```python
from build123d import *

# Parameters (mm, degrees)
SKETCH1_R           = 4.1
BOSS_EXTRUDE1_DEPTH = 10
SKETCH2_W           = 28.190778624
SKETCH2_H           = 5
BOSS_EXTRUDE2_DEPTH = 15
SKETCH4_R           = 2.6
CUT_EXTRUDE1_DEPTH  = 20
CHAMFER1_SIZE       = 15
SKETCH5_R           = 5.5
CUT_EXTRUDE2_DEPTH  = 20


with BuildPart() as part:
    # Sketch1 → Boss-Extrude1 (new body)
    with BuildSketch(Plane.XY):
        Polygon((535.624793848, 194.951481696), (535.624793848, 0), (507.434015224, 0), (507.434015224, 184.690877396), (497.173410925, 212.881656019), (525.364189548, 223.142260319), align=None)
        with Locations((516.399102386, 203.916568858)):
            Circle(SKETCH1_R, mode=Mode.SUBTRACT)
    extrude(amount=BOSS_EXTRUDE1_DEPTH)

    # Sketch2 → Boss-Extrude2 (add)
    with BuildSketch(Plane.XY.offset(10)):
        with Locations((521.529404536, 2.5)):
            Rectangle(SKETCH2_W, SKETCH2_H)
    extrude(amount=BOSS_EXTRUDE2_DEPTH)

    # Sketch4 → Cut-Extrude1 (cut)
    with BuildSketch(Plane(origin=(0, 5, 0), x_dir=(1, 0, 0), z_dir=(0, 1, 0))):
        with Locations(Location((528.577099192, -17.5, 0), (0, 0, 270))):
            Circle(SKETCH4_R)
        with Locations(Location((514.48170988, -17.5, 0), (0, 0, 270))):
            Circle(SKETCH4_R)
    extrude(amount=-CUT_EXTRUDE1_DEPTH, mode=Mode.SUBTRACT)

    # Chamfer1
    # the kernel refuses this chamfer: 15 mm, written as the material it adds along each edge
    with BuildSketch(Plane(origin=(535.624793848, 5, 10), x_dir=(0, 0.9996219169112968, -0.02749587661058632), z_dir=(-1, 0, 0))) as chamfer1_piece_1_section:
        Polygon((CHAMFER1_SIZE * 0.999621916911, -CHAMFER1_SIZE * 0.0274958766106), (-CHAMFER1_SIZE * 0.0274958766106, -CHAMFER1_SIZE * 0.999621916911), (0, 0), align=None)
    chamfer1_piece_1 = extrude(amount=28.190778624, mode=Mode.PRIVATE)
    chamfer1_piece_1 = split(chamfer1_piece_1, bisect_by=Plane(origin=(521.529400048, 10.087187588, 25), z_dir=(0, 0, -1)), keep=Keep.TOP, mode=Mode.PRIVATE)
    chamfer1_piece_1 = chamfer1_piece_1 - Plane(origin=(528.577099192, 10.087187588, 17.5), x_dir=(0, 0, 1), z_dir=(0, 1, 0)) * Cylinder(2.6, 117, mode=Mode.PRIVATE)
    chamfer1_piece_1 = chamfer1_piece_1 - Plane(origin=(514.48170988, 10.087187588, 17.5), x_dir=(0, 0, 1), z_dir=(0, 1, 0)) * Cylinder(2.6, 117, mode=Mode.PRIVATE)
    add(chamfer1_piece_1)

    # Sketch5 → Cut-Extrude2 (cut)
    with BuildSketch(Plane(origin=(0, 5, 0), x_dir=(1, 0, 0), z_dir=(0, 1, 0))):
        with Locations(Location((514.48170988, -17.5, 0), (0, 0, 270))):
            Circle(SKETCH5_R)
        with Locations(Location((528.577099192, -17.5, 0), (0, 0, 270))):
            Circle(SKETCH5_R)
    extrude(amount=CUT_EXTRUDE2_DEPTH, mode=Mode.SUBTRACT)


solid = part.part
```
Design review of the part built by this model. Coordinates are the model's own, in mm. A direction names the side the tool comes from. Give positions to 0.01 mm unless a question says otherwise; leave off trailing zeros. Order: outer loops, then holes, each group sorted by start corner. A loop starts at its lowest first (then second) coordinate and runs counter-clockwise, first axis right, second up. Notation, with made-up numbers: (-7, 56) - (21, 56) arc R27 cw to (21, 90) - close; hole circle Ø5 at (-3, 56). An arc over 180 degrees is marked (long way). Use a Markdown table: item, result. Add a question column.
(1) Add section B-B on y = 159. Give the boundary of the cut face in (x, z).
(2) Add section C-C on x = 504.5. Give the boundary of the cut face in (y, z), then the cut area to 3 significant figures.
(3) Clearance check with flat-ended pins moving along their axes: P1, Ø6, axis at x = 529, y = 81, coming from the +Z side; P2, Ø8, axis at x = 508.5, z = 11.5, coming from the +Y side; P3, Ø10, axis at x = 514.48, z = 17.5, coming from the +Y side. State where each tip first meets the part, or that it passes through.
(4) Add section A-A on z = 17.5. Give the boundary of the cut face in (x, y).
(5) Mouldability with a two-part tool opening along X and no side actions: class faces 1 (the face through (521, 123, 10)), 2 (the face through (514.724, 10.052, 12.005)), 3 (the face through (511.07, 217.94, 4.93)) as +X half, -X half, draft (parallel to the pull), parting line (faces both ways), or undercut.
(6) Wall thickness on probe 1 along X at (y, z) = (9.5, 17.5); probe 2 along X at (y, z) = (1.2, 17.5); probe 3 along Z at (x, y) = (532.5, 197.5): over which ranges is each line inside the solid? List them lowest first. Write a range as [from, to].
(7) Machinability: for faces 4 (the face through (527, 5, 20)), 5 (the face through (530.423, 209.244, 4.93)), 6 (the face through (507.434, 93, 4)), which of the approach directions +Z, -Z, +X, -X, +Y, -Y give a long, thin tool a straight path to every point of the face, cutting with its end or side? Answer none if there is none.
Report:
| question | item | result |
|---|---|---|
| 1 | outline | (507.43, 0) - (535.62, 0) - (535.62, 10) - (507.43, 10) - close |
| 2 | outline | (192.75, 0) - (215.55, 0) - (215.55, 10) - (192.75, 10) - close |
| 2 | area | 228 mm² |
| 3 | P1 | stops at z = 10 |
| 3 | P2 | stops at y = 218.35 |
| 3 | P3 | stops at y = 5 |
| 4 | outline | (507.43, 0) - (511.88, 0) - (511.88, 5) - (508.98, 5) - (508.98, 12.5) - (507.43, 12.5) - close; (517.08, 0) - (525.98, 0) - (525.98, 5) - (523.08, 5) - (523.08, 12.5) - (519.98, 12.5) - (519.98, 5) - (517.08, 5) - close; (531.18, 0) - (535.62, 0) - (535.62, 12.5) - (534.08, 12.5) - (534.08, 5) - (531.18, 5) - close |
| 5 | face 1 | draft |
| 5 | face 2 | undercut |
| 5 | face 3 | -X half |
| 6 | probe 1 | x = [507.43, 508.98], [519.98, 523.08], [534.08, 535.62] |
| 6 | probe 2 | x = [507.43, 511.88], [517.08, 525.98], [531.18, 535.62] |
| 6 | probe 3 | z = [0, 10] |
| 7 | face 4 | +Y |
| 7 | face 5 | +Z, -Z, +X, +Y |
| 7 | face 6 | +Z, -Z, -X, -Y |
